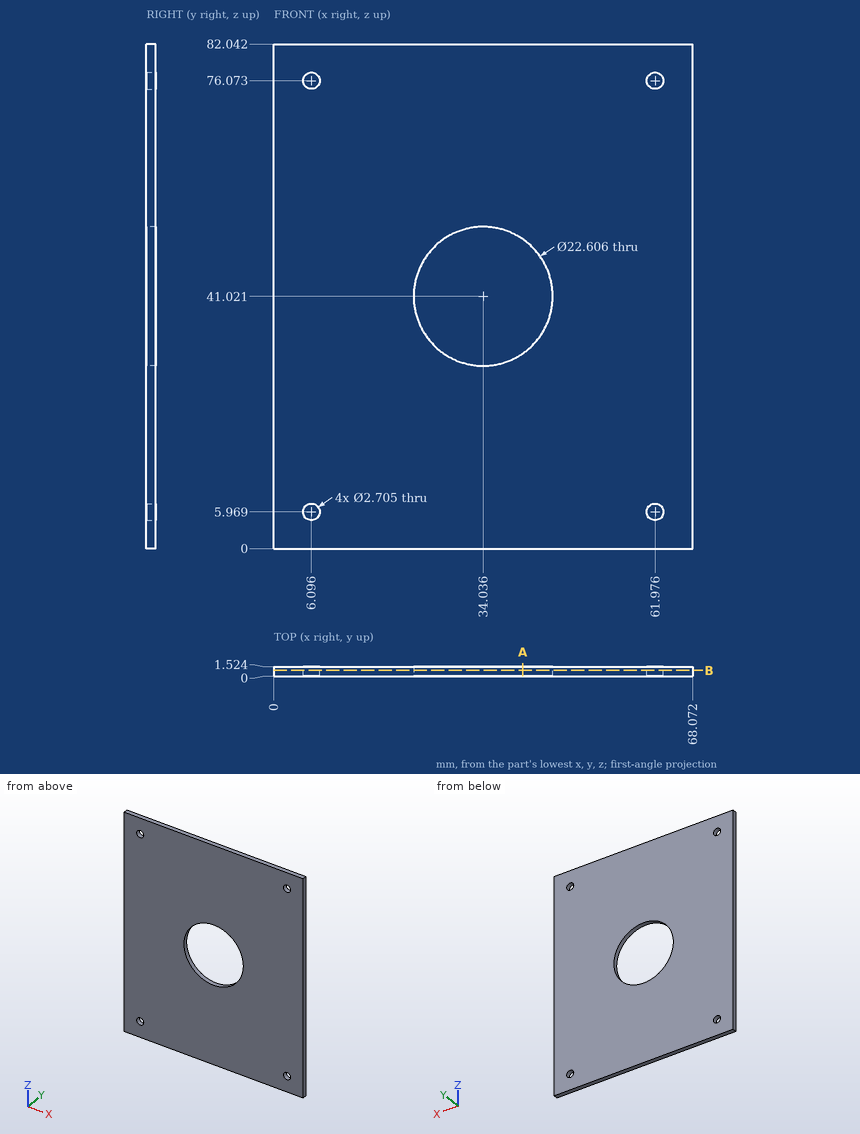
Can you work these out from the drawing? Everything is in mm from the part's minimum corner. Give positions to 0.01 mm unless a question says otherwise; leave off trailing zeros. Order: outer loops, then holes, each group sorted by start corner. A loop starts at its lowest first (then second) coordinate and runs counter-clockwise, first axis right, second up.
Item 1: I need wall thicknesses on line 1 (Z direction, x = 34.5, y = 0.7); line 2 (X direction, y = 0.3, z = 48.5); line 3 (Z direction, x = 39, y = 1). Which ranges of each line are inside material? Lowest first, please.
Item 2: If we section it at B-B, the plane y = 0.9: Write out the boundary of the cut face in (x, z) (1 decimal).
Item 3: If we section it at A-A, the plane x = 40.5: Write out the boundary of the cut face in (y, z).
Values:
1. line 1: z = 0 to 29.73, 52.31 to 82.04
1. line 2: x = 0 to 25.56, 42.51 to 68.07
1. line 3: z = 0 to 30.87, 51.18 to 82.04
2. outline: (0, 0) - (68.1, 0) - (68.1, 82) - (0, 82) - close; hole circle Ø2.7 at (6.1, 6); hole circle Ø2.7 at (6.1, 76.1); hole circle Ø22.6 at (34, 41); hole circle Ø2.7 at (62, 6); hole circle Ø2.7 at (62, 76.1)
3. outline: (0, 0) - (1.52, 0) - (1.52, 31.75) - (0, 31.75) - close; (0, 50.29) - (1.52, 50.29) - (1.52, 82.04) - (0, 82.04) - close
